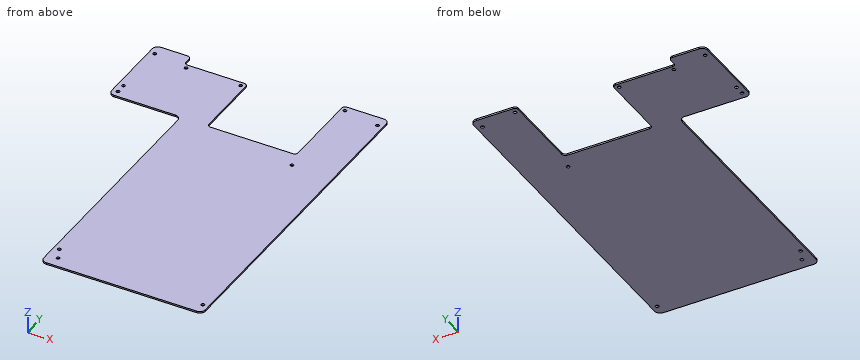
Autodesk Inventor part; units mm, degrees
ref_plane "YZ Plane" through (0, 0, 0) normal (1, 0, 0) x (0, 1, 0)
ref_plane "XZ Plane" through (0, 0, 0) normal (0, 1, 0) x (-1, 0, 0)
ref_plane "XY Plane" through (0, 0, 0) normal (0, 0, 1) x (1, 0, 0)
sketch "スケッチ2" plane through (0, 0, 0) normal (0, 0, 1) x (1, 0, 0)
  line L0 (-75, 37.5) -> (75, 37.5)
  line L1 (80, 32.5) -> (80, -257.5)
  line L2 (75, -262.5) -> (-60, -262.5)
  line L3 (-65, -183.2657) -> (-65, -42.5)
  arc A0 (80, 32.5) -> (75, 37.5) centre (75, 32.5) ccw
  arc A1 (75, -262.5) -> (80, -257.5) centre (75, -257.5) ccw
  line L4 (-65, -257.5) -> (-65, -183.1423)
  arc A2 (-65, -257.5) -> (-60, -262.5) centre (-60, -257.5) ccw
  line L5 (-75, 37.5) -> (-125, 37.5)
  line L6 (-130, 32.5) -> (-130, -32.5)
  line L7 (-125, -37.5) -> (-70, -37.5)
  arc A3 (-125, 37.5) -> (-130, 32.5) centre (-125, 32.5) ccw
  arc A4 (-130, -32.5) -> (-125, -37.5) centre (-125, -32.5) ccw
  arc A5 (-65, -42.5) -> (-70, -37.5) centre (-70, -42.5) ccw
  point P0 (0, 0)
  point P1 (-75, 37.5)
  point P2 (80, -262.5)
  point P3 (80, 37.5)
  point P4 (-65, -262.5)
  point P5 (-75, 0)
  point P6 (0, 37.5)
  point P7 (0, 0)
  point P8 (-130, 0)
  dimension "d1" = 300
  dimension "d24" = 5
  dimension "d49" = 210
  dimension "d50" = 5
  dimension "d51" = 75
  dimension "d78" = 145
extrude "押し出し1" add sketch "スケッチ2" along normal blind 1.5
sketch "スケッチ5" plane through (0, 0, 1.5) normal (0, 0, 1) x (1, 0, 0)
  line L0 (75, 37.5) -> (-125, 37.5)
  line L1 (80, -257.5) -> (80, 32.5)
  line L2 (-60, -262.5) -> (75, -262.5)
  line L3 (-130, 32.5) -> (-130, -32.5)
  line L4 (-125, -37.5) -> (-70, -37.5)
  line L5 (-65, -42.5) -> (-65, -257.5)
  point P0 (-125, 27.5)
  point P1 (75, 27.5)
  point P2 (75, -252.5)
  point P3 (-70, 37.5)
  point P4 (-125, -31.5)
  point P5 (-60, -241.5)
  point P6 (43, -52.5)
  point P7 (43, 32.5)
  point P8 (-45, 22.5)
  point P9 (-125, -22.5)
  point P10 (-55, -252.5)
  point P11 (-94, 22.5)
  dimension "d25" = 10
  dimension "d27" = 5
  dimension "d44" = 80
  dimension "d46" = 85
  dimension "d52" = 5
  dimension "d55" = 10
  dimension "d56" = 10
  dimension "d58" = 21
  dimension "d59" = 5
  dimension "d60" = 15
  dimension "d61" = 69
  dimension "d62" = 5
  dimension "d66" = 54
  dimension "d67" = 49
  dimension "d77" = 37
hole "穴3" at (-125, 27.5, 1.5) at (75, 27.5, 1.5) at (75, -252.5, 1.5) at (-125, -31.5, 1.5) at (-60, -241.5, 1.5) at (-45, 22.5, 1.5) at (43, 32.5, 1.5) at (43, -52.5, 1.5) at (-125, -22.5, 1.5) at (-55, -252.5, 1.5) at (-94, 22.5, 1.5) direction (0, 0, -1) diameter 3 depth 8.1 tip angle 118
sketch "スケッチ6" plane through (0, 0, 1.5) normal (0, 0, 1) x (1, 0, 0)
  point P0 (0, 0)
sketch "スケッチ7" plane through (0, 0, 1.5) normal (0, 0, 1) x (1, 0, 0)
  line L0 (-41, 26.5) -> (-98, 26.5)
  line L1 (-98, 26.5) -> (-98, 37.5)
  line L2 (-98, 37.5) -> (39, 37.5)
  line L3 (39, 37.5) -> (39, -38.5)
  line L4 (-41, 0) -> (-41, 26.5)
  circle A0 centre (-45, 22.5) radius 1.5
  circle A1 centre (-94, 22.5) radius 1.5
  line L5 (75, 37.5) -> (-125, 37.5)
  line L6 (39, -38.5) -> (-41, -38.5)
  line L7 (-41, -38.5) -> (-41, 0)
  point P0 (-25.5, 0)
  dimension "d68" = 4
  dimension "d69" = 4
  dimension "d70" = 4
  dimension "d74" = 76
  dimension "d75" = 80
extrude "押し出し2" cut sketch "スケッチ7" against normal blind 10 contours L0 L1 L2 L3 L6 L7 L4
fillet "フィレット1" radius 3 6 edges at (-98, 26.5, 0.75) (-41, 26.5, 0.75) (-98, 37.5, 0.75) (-41, -38.5, 0.75) (39, -38.5, 0.75) (39, 37.5, 0.75)
properties part number "天板"
Part model, mm, in its own coordinate system. Coordinates: 2 decimals unless noted, no trailing zeros. Order: outer loops, then holes, each group sorted by start corner. A loop starts at its lowest first (then second) coordinate and runs counter-clockwise, first axis right, second up.
(1) Probe L1, parallel to Y at x = 43, z = 0.45; L2, parallel to X at y = 22.5, z = 1; L3, parallel to X at y = -252.5, z = 1.1. List the from-to ranges inside material, lowest first.
Check sheet entries:
L1: y = -262.5 to -54, -51 to 31, 34 to 37.5
L2: x = -130 to -95.5, -92.5 to -46.5, -43.5 to -41, 39 to 80
L3: x = -65 to -56.5, -53.5 to 73.5, 76.5 to 80
(2) Slice it at C-C, the plane z = 1.15. State how many separate pieces and enclosed holes the cut face has, and give its area (3 significant figures).
Check sheet entries:
separate pieces: 1
enclosed holes: 11
area: 41,600 mm2
(3) Pin check, flat tip, straight feed: pin 1 Ø5 at (x, y) = (-125, 27.5) entering from +Z. Stop position of the tip, or through.
Check sheet entries:
pin 1: stops at z = 1.5
(4) Slice it at D-D, the plane x = -7. Write the cut outline in (y, z), and give its area (3 significant figures).
Check sheet entries:
outline: (-262.5, 0) - (-38.5, 0) - (-38.5, 1.5) - (-262.5, 1.5) - close
area: 336 mm2
(5) Slice it at B-B, the plane y = -195. Write the cut outline in (x, z), and give its area (4 significant figures).
Check sheet entries:
outline: (-65, 0) - (80, 0) - (80, 1.5) - (-65, 1.5) - close
area: 217.5 mm2
(6) Slice it at A-A, the plane y = 0.5. Write the cut outline in (x, z).
Check sheet entries:
outline: (-130, 0) - (-41, 0) - (-41, 1.5) - (-130, 1.5) - close; (39, 0) - (80, 0) - (80, 1.5) - (39, 1.5) - close
